Input: dimensioned drawing with shaded views. Units: mm. Origin: part minimum x, y, z. Give positions to 0.01 mm unless a question says otherwise; leave off trailing zeros. Loops run counter-clockwise (first coordinate to the right, second up) from the corner with the lowest first, then second, coordinate; pieces in that order, holes last. Notation, with made-up numbers: M 51,2 L 77,2 A9 ccw 77,17 Z; hole C 35,31.25 d6. An arc over 180 degrees is marked long. Answer in a Markdown table with one row per item.
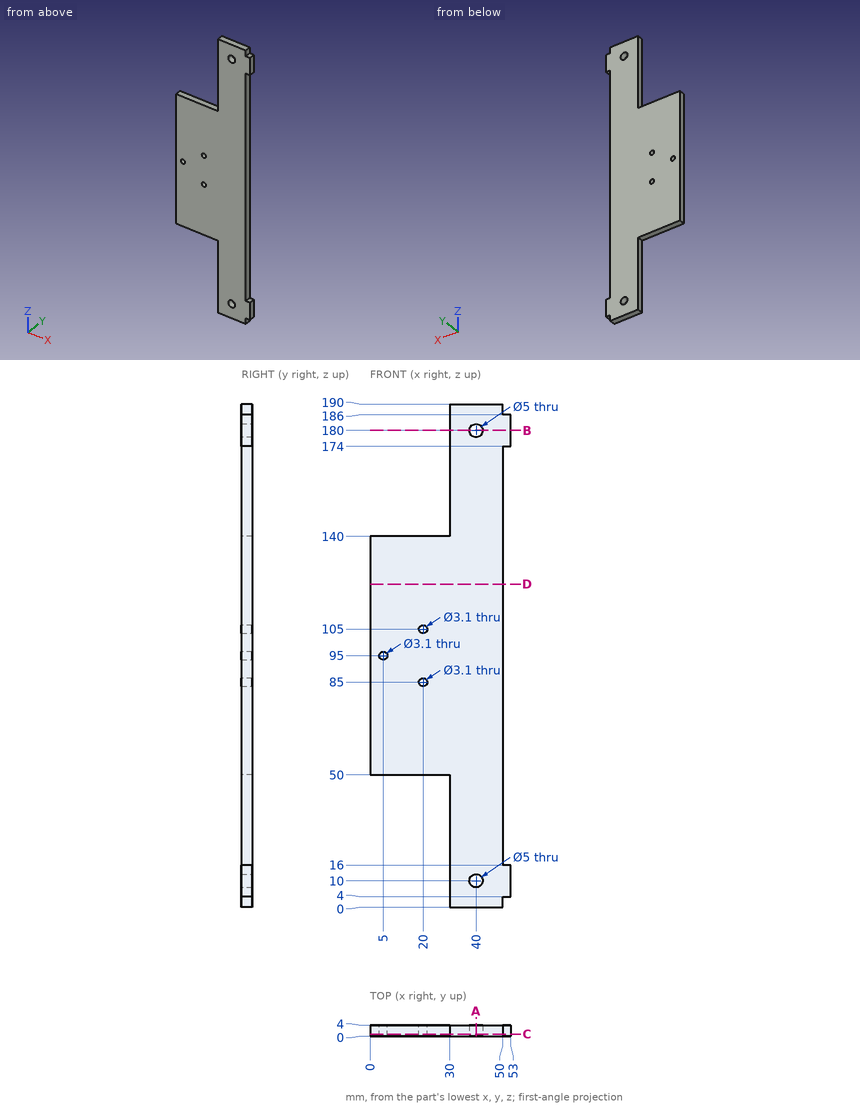
Q1. Section query A-A (x = 40). Output: boundary loops of the cut face in (y, z), plus the area to 3 significant figures.
Values follow:
| item | result |
|---|---|
| outline | M 0,0 L 4,0 L 4,7.5 L 0,7.5 Z; M 0,12.5 L 4,12.5 L 4,177.5 L 0,177.5 Z; M 0,182.5 L 4,182.5 L 4,190 L 0,190 Z |
| area | 720 mm^2 |
Q2. Ray query, probe 1 along X at (y, z) = (0.8, 10); probe 2 along X at (y, z) = (1.7, 85); probe 3 along X at (y, z) = (0.8, 124.5). Return the intervals inside material, ascending. Write a range as from..to.
Values follow:
| item | result |
|---|---|
| probe 1 | 30..37.5, 42.5..53 |
| probe 2 | 0..18.45, 21.55..50 |
| probe 3 | 0..50 |
Q3. Section query D-D (z = 122). Output: boundary loops of the cut face in (x, y).
Values follow:
| item | result |
|---|---|
| outline | M 0,0 L 50,0 L 50,4 L 0,4 Z |
Q4. Section query B-B (z = 180). Output: boundary loops of the cut face in (x, y), plus the area to 3 significant figures.
Values follow:
| item | result |
|---|---|
| outline | M 30,0 L 37.5,0 L 37.5,4 L 30,4 Z; M 42.5,0 L 53,0 L 53,4 L 42.5,4 Z |
| area | 72.0 mm^2 |
Q5. Section query C-C (y = 0.75). Output: boundary loops of the cut face in (x, z), plus the area to 3 significant figures.
Values follow:
| item | result |
|---|---|
| outline | M 0,50 L 30,50 L 30,0 L 50,0 L 50,4 L 53,4 L 53,16 L 50,16 L 50,174 L 53,174 L 53,186 L 50,186 L 50,190 L 30,190 L 30,140 L 0,140 Z; hole C 5,95 d3.1; hole C 20,85 d3.1; hole C 20,105 d3.1; hole C 40,10 d5; hole C 40,180 d5 |
| area | 6,510 mm^2 |
Q6. Contact query for flat-ended pins moving along their axis: pin 1 Ø1 at (y, z) = (1, 28) entering from +X; pin 2 Ø0.9 at (x, y) = (51.5, 1.5) entering from -Z; pin 3 Ø1.5 at (x, y) = (51, 2.5) entering from +Z. Output: stop coordinate, or through.
Values follow:
| item | result |
|---|---|
| pin 1 | x = 50 |
| pin 2 | z = 4 |
| pin 3 | z = 186 |
